Source: three-view drawing plus pictorial views. Frame: mm from the lowest corner of the part. A direction names the side the tool comes from. Give positions to 0.01 mm unless a question says otherwise; leave off trailing zeros. Write each loop counter-clockwise with the first axis right and the second up, starting at its lowest first coordinate (ties: lowest second). Pieces come first, ordered by that corner, then holes. Notation, with made-up numbers: M 42,53 L 95,53 A26 ccw 95,81 Z; hole C 19,0.25 d8. An arc over 180 degrees is marked long. Return JSON: item names as keys, results as strings.
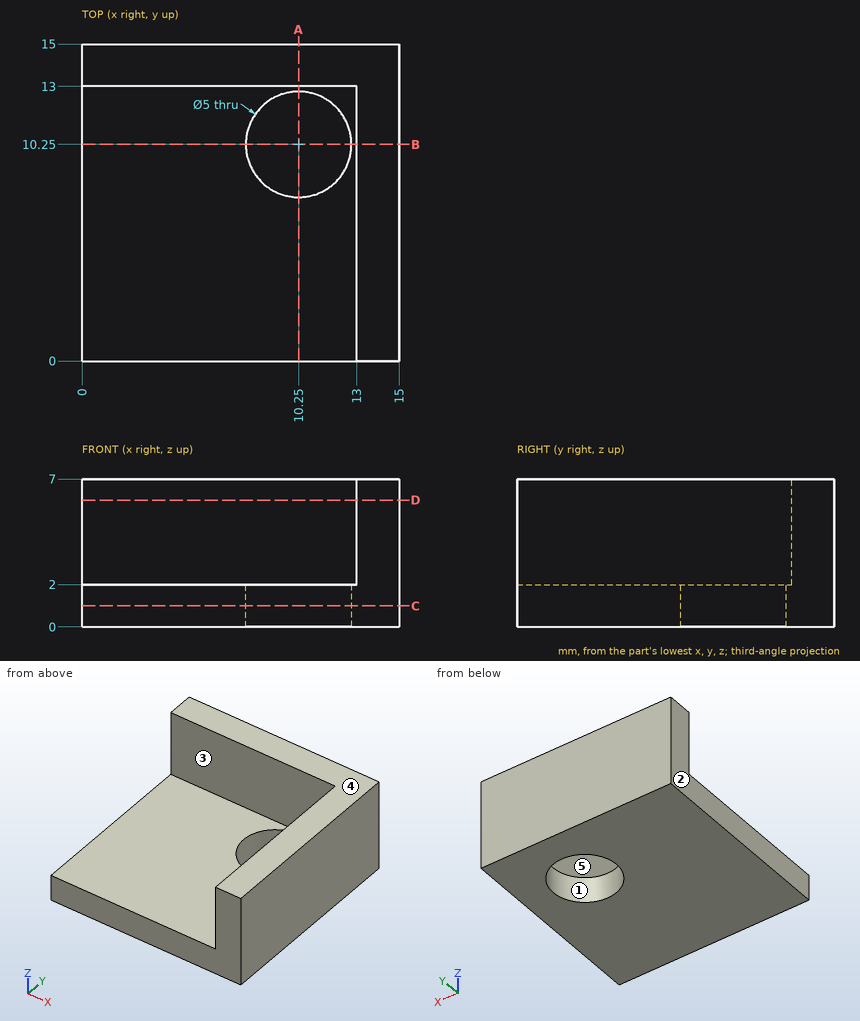
1) Cut plane C-C, the plane z = 1. Return the cut outline in (x, y), then the cut area to 3 significant figures.
Numbers:
{"outline": "M 0,0 L 15,0 L 15,15 L 0,15 Z; hole C 10.25,10.25 d5", "area": "205 mm²"}
2) Set-up query: the marked faces 4 and 5. Return all of +Z, -Z, +X, -X, +Y, -Y with unobstructed straight access to the full face (end or side cutting, diameter ignored); none if empty.
Numbers:
{"face 4": "+Z, +X, -X, +Y, -Y", "face 5": "+Z, -X, -Y"}
3) Draft query along Y for the marked faces 1, 2 and 3. Return one class per face: released by +Y, released by -Y, zero draft, split by the parting line, or undercut.
Numbers:
{"face 1": "undercut", "face 2": "zero draft", "face 3": "released by -Y"}
4) Cut plane A-A, the plane x = 10.25. Return the cut outline in (y, z), then the cut area to 3 significant figures.
Numbers:
{"outline": "M 0,0 L 7.75,0 L 7.75,2 L 0,2 Z; M 12.75,0 L 15,0 L 15,7 L 13,7 L 13,2 L 12.75,2 Z", "area": "30.0 mm²"}
5) Contact query for flat-ended pins moving along their axis: pin 1 Ø1.5 at (x, z) = (2, 6) entering from -Y; pin 2 Ø2.5 at (y, z) = (8.5, 3.5) entering from -X; pin 3 Ø6.5 at (x, y) = (5, 9.5) entering from +Z. Output: stop coordinate, or through.
Numbers:
{"pin 1": "stops at y = 13", "pin 2": "stops at x = 13", "pin 3": "stops at z = 2"}
6) Cut plane D-D, the plane z = 6. Return the cut outline in (x, y), then the cut area to 3 significant figures.
Numbers:
{"outline": "M 0,13 L 13,13 L 13,0 L 15,0 L 15,15 L 0,15 Z", "area": "56.0 mm²"}
7) Line query: line 1 (Y direction, x = 10.25, z = 1.5); line 2 (Z direction, x = 11, y = 1.75); line 3 (X direction, y = 10.25, z = 3.75). Output: solid intervals per line, ascending. Write a range as [from, to].
Numbers:
{"line 1": "y = [0, 7.75], [12.75, 15]", "line 2": "z = [0, 2]", "line 3": "x = [13, 15]"}
